Geometry check sheet. Reference: the model listing, model coordinates, mm. A direction names the side the tool comes from. Round coordinates to 2 decimals unless told otherwise and drop trailing zeros. Write each loop counter-clockwise with the first axis right and the second up, starting at its lowest first coordinate (ties: lowest second). Pieces come first, ordered by that corner, then holes. Notation, with made-up numbers: (79.25, 47.5) -> (98.25, 47.5) arc R34 ccw to (98.25, 81.5) -> close; hole circle Ø10 at (89.5, 71). An arc over 180 degrees is marked (long way). Return JSON: item names as keys, results as strings. Group by question number.
from build123d import *

# Parameters (mm, degrees)
SKETCH1_W           = 80
SKETCH1_H           = 70
SKETCH1_R           = 2.4
BOSS_EXTRUDE1_DEPTH = 6.35
FILLET1_R           = 10


with BuildPart() as part:
    # Sketch1 → Boss-Extrude1 (new body)
    with BuildSketch(Plane(origin=(0, 0, 0), x_dir=(1, 0, 0), z_dir=(0, 1, 0))):
        Rectangle(SKETCH1_W, SKETCH1_H)
        with Locations((0, 18)):
            Circle(SKETCH1_R, mode=Mode.SUBTRACT)
        with Locations((0, -5.7)):
            Circle(SKETCH1_R, mode=Mode.SUBTRACT)
        with Locations((0, -29.4)):
            Circle(SKETCH1_R, mode=Mode.SUBTRACT)
        Polygon((-20, -35), (-10, -35), (-10.5, -40.715), (-19.5, -40.715), align=None)
        Polygon((10, -35), (10.5, -40.715), (19.5, -40.715), (20, -35), align=None)
        Polygon((-35, -35), (-25, -35), (-25.5, -40.715), (-34.5, -40.715), align=None)
        Polygon((25, -35), (25.5, -40.715), (34.5, -40.715), (35, -35), align=None)
    extrude(amount=BOSS_EXTRUDE1_DEPTH)

    # Fillet1
    fillet1_edges = [part.edges().sort_by_distance(p)[0] for p in [
        (-40, 3.175, -35),
        (40, 3.175, -35),
    ]]
    fillet(fillet1_edges, radius=FILLET1_R)


solid = part.part
1) Tool access check on faces 5 (the face through (22, 3, 35)), 6 (the face through (-40, 3, 5)), 7 (the face through (37, 3, 35)), 8 (the face through (-38, 3, 35)). Record the directions out of +Z, -Z, +X, -X, +Y, -Y that give a thin tool (end or side, any length) a straight path to the whole face; none if there is none.
2) Sectioned sample at D-D on z = -19.5. Enter the section's corners in (x, y), and give its area (3 significant figures).
3) Sectioned sample at B-B on x = 0. Enter the section's corners in (y, z).
4) Mould release check, pull along Z, two halves, no side actions. Record for faces 1 (the face through (1.29, 3.131, 3.676)), 2 (the face through (0, 3, 27)), 3 (the face through (40, 3, 5)), 4 (the face through (19.746, 3.131, 37.898)): +Z half, -Z half, draft (parallel to the pull), parting line (faces both ways), or undercut.
5) Sectioned sample at C-C on y = 2.5. Enter the section's corners in (x, z) (3 decimals).
6) Sectioned sample at A-A on z = 29.4. Enter the section's corners in (x, y).
7) Material ranges on probe 1 along Z at (x, y) = (0, 3.75); probe 2 along X at (y, z) = (3.5, -18); probe 3 along Z at (x, y) = (-22, 1.5), recorded low to high. Write a range as [from, to].
Evaluation:
{
 "1": {"face 5": "+Z, +Y, -Y", "face 6": "+Z, -Z, -X, +Y, -Y", "face 7": "+Z, +X, +Y, -Y", "face 8": "+Z, -X, +Y, -Y"},
 "2": {"outline": "(-40, 0) -> (-1.87, 0) -> (-1.87, 6.35) -> (-40, 6.35) -> close; (1.87, 0) -> (40, 0) -> (40, 6.35) -> (1.87, 6.35) -> close", "area": "484 mm2"},
 "3": {"outline": "(0, -35) -> (6.35, -35) -> (6.35, -20.4) -> (0, -20.4) -> close; (0, -15.6) -> (6.35, -15.6) -> (6.35, 3.3) -> (0, 3.3) -> close; (0, 8.1) -> (6.35, 8.1) -> (6.35, 27) -> (0, 27) -> close; (0, 31.8) -> (6.35, 31.8) -> (6.35, 35) -> (0, 35) -> close"},
 "4": {"face 1": "undercut", "face 2": "undercut", "face 3": "draft", "face 4": "+Z half"},
 "5": {"outline": "(-40, -25) arc R10 ccw to (-30, -35) -> (30, -35) arc R10 ccw to (40, -25) -> (40, 35) -> (35, 35) -> (34.5, 40.715) -> (25.5, 40.715) -> (25, 35) -> (20, 35) -> (19.5, 40.715) -> (10.5, 40.715) -> (10, 35) -> (-10, 35) -> (-10.5, 40.715) -> (-19.5, 40.715) -> (-20, 35) -> (-25, 35) -> (-25.5, 40.715) -> (-34.5, 40.715) -> (-35, 35) -> (-40, 35) -> close; hole circle Ø4.8 at (0, -18); hole circle Ø4.8 at (0, 5.7); hole circle Ø4.8 at (0, 29.4)"},
 "6": {"outline": "(-40, 0) -> (-2.4, 0) -> (-2.4, 6.35) -> (-40, 6.35) -> close; (2.4, 0) -> (40, 0) -> (40, 6.35) -> (2.4, 6.35) -> close"},
 "7": {"probe 1": "z = [-35, -20.4], [-15.6, 3.3], [8.1, 27], [31.8, 35]", "probe 2": "x = [-40, -2.4], [2.4, 40]", "probe 3": "z = [-35, 35]"}
}
